The model under review builds one solid part; all positions refer to its coordinate system, in mm. A direction names the side the tool comes from. Coordinates: 2 decimals unless noted, no trailing zeros. Order: outer loops, then holes, each group sorted by start corner. A loop starts at its lowest first (then second) coordinate and runs counter-clockwise, first axis right, second up. Notation, with made-up numbers: M 10.5,16 L 27.5,16 A23 cw 27.5,49 Z; hole C 44,-15 d1. An arc over 180 degrees is marked long. Write each question's results on one line, items separated by ' | '.
from build123d import *

# Parameters (mm, degrees)
F0_W     = 105.3
F0_H     = 75.3
F1_DEPTH = 2
F2_DEPTH = 6.7
F3_R     = 3.5
F3_R_2   = 2.1
F4_DEPTH = 3
F5_DEPTH = 25


with BuildPart() as f1:
    # F0 (on Top) → F1 (new body)
    with BuildSketch(Plane.XY):
        with BuildLine():
            Line((52.65, 39.65), (-52.65, 39.65))
            ThreePointArc((-52.65, 39.65), (-54.0642135624, 39.0642135624), (-54.65, 37.65))
            Line((-54.65, 37.65), (-54.65, -37.65))
            ThreePointArc((-54.65, -37.65), (-54.0642135624, -39.0642135624), (-52.65, -39.65))
            Line((-52.65, -39.65), (52.65, -39.65))
            ThreePointArc((52.65, -39.65), (54.0642135624, -39.0642135624), (54.65, -37.65))
            Line((54.65, -37.65), (54.65, 37.65))
            ThreePointArc((54.65, 37.65), (54.0642135624, 39.0642135624), (52.65, 39.65))
        make_face()
        Rectangle(F0_W, F0_H, mode=Mode.SUBTRACT)
        Rectangle(F0_W, F0_H)
    extrude(amount=F1_DEPTH)

    # F0 (on Top) → F2 (join)
    with BuildSketch(Plane.XY):
        with BuildLine():
            Line((52.65, 39.65), (-52.65, 39.65))
            ThreePointArc((-52.65, 39.65), (-54.0642135624, 39.0642135624), (-54.65, 37.65))
            Line((-54.65, 37.65), (-54.65, -37.65))
            ThreePointArc((-54.65, -37.65), (-54.0642135624, -39.0642135624), (-52.65, -39.65))
            Line((-52.65, -39.65), (52.65, -39.65))
            ThreePointArc((52.65, -39.65), (54.0642135624, -39.0642135624), (54.65, -37.65))
            Line((54.65, -37.65), (54.65, 37.65))
            ThreePointArc((54.65, 37.65), (54.0642135624, 39.0642135624), (52.65, 39.65))
        make_face()
        Rectangle(F0_W, F0_H, mode=Mode.SUBTRACT)
    extrude(amount=F2_DEPTH)

    # F3 (on face) → F4 (join)
    with BuildSketch(Plane.XY.offset(2)):
        with Locations((-48, 33)):
            Circle(F3_R)
        with Locations((-48, 33)):
            Circle(F3_R_2, mode=Mode.SUBTRACT)
        with Locations((48, 33)):
            Circle(F3_R)
        with Locations((48, 33)):
            Circle(F3_R_2, mode=Mode.SUBTRACT)
        with Locations((48, -33)):
            Circle(F3_R)
        with Locations((48, -33)):
            Circle(F3_R_2, mode=Mode.SUBTRACT)
        with Locations((-48, -33)):
            Circle(F3_R)
        with Locations((-48, -33)):
            Circle(F3_R_2, mode=Mode.SUBTRACT)
    extrude(amount=F4_DEPTH)

    # F5 (cut): faces of the model
    f5_faces = [f1.faces().sort_by_distance(p)[0] for p in [
        (-48, 33, 2),
        (48, 33, 2),
        (48, -33, 2),
        (-48, -33, 2),
    ]]
    extrude(f5_faces, amount=-F5_DEPTH, mode=Mode.SUBTRACT)


solid = f1.part
1) For pin 1 (5 mm diameter, centred on x = 48, y = 33, fed in from +Z); pin 2 (5 mm diameter, centred on x = 48, y = -33, fed in from -Z); pin 3 (3 mm diameter, centred on x = -11, y = -28.5, fed in from +Z), all flat-tipped, find the tip position at first contact; note any pin that passes through.
Solutions:
pin 1: z = 5 | pin 2: z = 0 | pin 3: z = 2
2) Take a section at D-D on x = -17.5. State the section outline as (y, z) points, plus the area to 3 significant figures.
Solutions:
outline: M -39.65,0 L 39.65,0 L 39.65,6.7 L 37.65,6.7 L 37.65,2 L -37.65,2 L -37.65,6.7 L -39.65,6.7 Z | area: 177 mm2
3) To check wall thickness, follow line 1 along Y through (x, z) = (-48, 1.35); line 2 along Y through (x, z) = (48, 3.4); line 3 along Y through (x, z) = (-16.5, 4.75). State the ranges of each line that lie inside material, in increasing order.
Solutions:
line 1: -39.65 to -35.1, -30.9 to 30.9, 35.1 to 39.65 | line 2: -39.65 to -37.65, -36.5 to -35.1, -30.9 to -29.5, 29.5 to 30.9, 35.1 to 36.5, 37.65 to 39.65 | line 3: -39.65 to -37.65, 37.65 to 39.65
4) Take a section at B-B on x = 48. State the section outline as (y, z) points.
Solutions:
outline: M -39.65,0 L -35.1,0 L -35.1,5 L -36.5,5 L -36.5,2 L -37.65,2 L -37.65,6.7 L -39.65,6.7 Z; M -30.9,0 L 30.9,0 L 30.9,5 L 29.5,5 L 29.5,2 L -29.5,2 L -29.5,5 L -30.9,5 Z; M 35.1,0 L 39.65,0 L 39.65,6.7 L 37.65,6.7 L 37.65,2 L 36.5,2 L 36.5,5 L 35.1,5 Z
5) For faces 1 (the flat face through (-54.65, 1, 3)), 2 (the flat face through (-1, -37.65, 4)), list the 3-axis set-ups (+Z, -Z, +X, -X, +Y, -Y) from which the entire face can be reached by the end or side of a thin tool; tool diameter is ignored.
Solutions:
face 1: +Z, -Z, -X, +Y, -Y | face 2: +Z
6) Take a section at A-A on z = 3.25. Count the separate pieces of the cut face and the enclosed holes in it, plus the area to 3 significant figures.
Solutions:
separate pieces: 5 | enclosed holes: 5 | area: 833 mm2
7) The part is to be moulded in two halves that separate along Y. For faces 3 (the flat face through (52.65, -1, 4)), 4 (the flat face through (-1, 1, 0)), 5 (the flat face through (1, 39.65, 3)), 6 (the cylindrical face through (-50.58, 35.365, 3.479)), say which applies: pulls with the +Y half, pulls with the -Y half, needs draft (parallel to the pull), parting line crosses it, or undercut.
Solutions:
face 3: undercut | face 4: needs draft | face 5: pulls with the +Y half | face 6: undercut
8) Take a section at C-C on y = 33. State the section outline as (x, z) points, plus the area to 3 significant figures.
Solutions:
outline: M -54.65,0 L -50.1,0 L -50.1,5 L -51.5,5 L -51.5,2 L -52.65,2 L -52.65,6.7 L -54.65,6.7 Z; M -45.9,0 L 45.9,0 L 45.9,5 L 44.5,5 L 44.5,2 L -44.5,2 L -44.5,5 L -45.9,5 Z; M 50.1,0 L 54.65,0 L 54.65,6.7 L 52.65,6.7 L 52.65,2 L 51.5,2 L 51.5,5 L 50.1,5 Z | area: 237 mm2
